Source: CAD feature listing. Evaluate the final solid. Frame: model axes, mm. Give positions to 0.01 mm unless a question says otherwise; leave off trailing zeros. Order: outer loops, then holes, each group sorted by start corner. A loop starts at its lowest first (then second) coordinate and runs counter-clockwise, first axis right, second up. Notation, with made-up numbers: M 60,77.25 L 103,77.25 A19 ccw 103,94.25 Z; hole C 87.25,-7 d10. An arc over 180 degrees is marked long. Answer in a Markdown table with one row per item. Add a question column.
(1) Section query C-C, the plane z = 0.8. Count the separate pieces of the cut face and the enclosed holes in it, plus the area to 3 significant figures.
(2) Section query A-A, the plane x = 0. Return loops of the section in (y, z).
(3) Pin query (flat end, axial travel): P1, Ø1.5, axis at x = 47.5, z = 1.5, coming from the -Y side; P2, Ø1.5, axis at y = 21, z = 3.5, coming from the -X side; P3, Ø1.5, axis at x = 48, z = 2, coming from the +Y side. Return the tip coordinate at first contact, or that it passes through.
(4) Section query D-D, the plane y = 31. Return loops of the section in (x, z).
(5) Section query B-B, the plane y = 10.16. Return loops of the section in (x, z).
(6) Material intervals for line 1 along Y through (x, z) = (-24, 1.7); line 2 along Y through (x, z) = (0, 1.2); line 3 along X through (y, z) = (3, 3.5), sorted ascending.
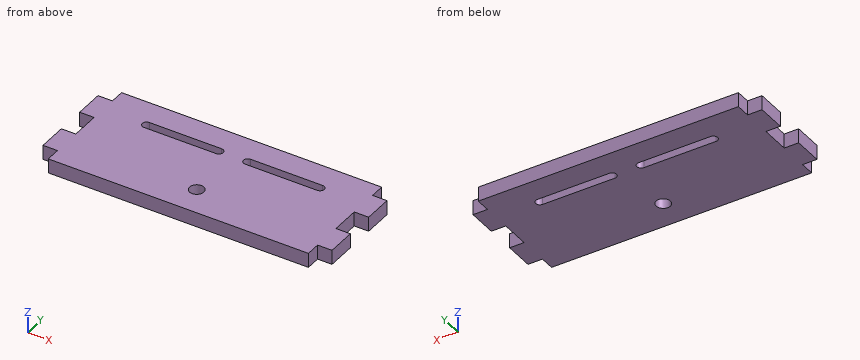
Autodesk Inventor part; units mm, degrees
ref_plane "YZ Plane" through (0, 0, 0) normal (1, 0, 0) x (0, 1, 0)
ref_plane "XZ Plane" through (0, 0, 0) normal (0, 1, 0) x (-1, 0, 0)
ref_plane "XY Plane" through (0, 0, 0) normal (0, 0, 1) x (1, 0, 0)
sketch "Sketch1" plane through (0, 0, 0) normal (0, 0, 1) x (1, 0, 0)
  line L0 (45.72, 0) -> (45.72, 40.64)
  line L1 (45.72, 40.64) -> (-45.72, 40.64)
  line L2 (-45.72, 40.64) -> (-45.72, 9.301)
  line L3 (-45.72, 5.08) -> (-50.8, 5.08)
  line L4 (-50.8, 5.08) -> (-50.8, 15.24)
  line L5 (-50.8, 15.24) -> (-45.72, 15.24)
  line L6 (-45.72, 15.24) -> (-45.72, 5.08)
  line L7 (-45.72, 25.4) -> (-50.8, 25.4)
  line L8 (-50.8, 25.4) -> (-50.8, 35.56)
  line L9 (-50.8, 35.56) -> (-45.72, 35.56)
  line L10 (-45.72, 35.56) -> (-45.72, 25.4)
  line L11 (-45.72, 45.72) -> (-50.8, 45.72)
  line L12 (-50.8, 45.72) -> (-50.8, 55.88)
  line L13 (-50.8, 55.88) -> (-45.72, 55.88)
  line L14 (-45.72, 55.88) -> (-45.72, 45.72)
  line L15 (0, 40.64) -> (0, 0) construction
  line L16 (45.72, 40.64) -> (45.72, 0)
  line L17 (45.72, 5.08) -> (50.8, 5.08)
  line L18 (50.8, 5.08) -> (50.8, 15.24)
  line L19 (50.8, 15.24) -> (45.72, 15.24)
  line L20 (45.72, 15.24) -> (45.72, 5.08)
  line L21 (45.72, 25.4) -> (50.8, 25.4)
  line L22 (50.8, 25.4) -> (50.8, 35.56)
  line L23 (50.8, 35.56) -> (45.72, 35.56)
  line L24 (45.72, 35.56) -> (45.72, 25.4)
  line L25 (45.72, 45.72) -> (50.8, 45.72)
  line L26 (50.8, 45.72) -> (50.8, 55.88)
  line L27 (50.8, 55.88) -> (45.72, 55.88)
  line L28 (45.72, 55.88) -> (45.72, 45.72)
  line L29 (-45.72, 5.08) -> (-45.72, 0)
  line L30 (-45.72, 0) -> (45.72, 0)
  line L31 (45.72, 40.64) -> (-45.72, 40.64)
  line L32 (-45.72, 40.64) -> (-45.72, 0)
  line L33 (-45.72, 0) -> (45.72, 0)
  line L34 (45.72, 0) -> (45.72, 40.64)
  dimension "d0" = 91.44
  dimension "d2" = 10.16
  dimension "d3" = 5.08
  dimension "d7" = 20.32
  dimension "d14" = 5.08
  dimension "d15" = 40.64
extrude "Extrusion2" add sketch "Sketch1" along normal blind 5.08 contours L30 L29 L6 L2 L1 L0 | L0 L19 L18 L17 | L3 L4 L5 L2 L6 | L0 L23 L22 L21 | L7 L8 L9 L2
sketch "Sketch4" plane through (0, 0, 5.08) normal (0, 0, 1) x (1, 0, 0)
  line L0 (45.72, 40.64) -> (-45.72, 40.64) construction
  line L1 (-30.48, 30.48) -> (-5.08, 30.48)
  line L2 (-30.48, 28.98) -> (-5.08, 28.98)
  line L3 (-5.08, 31.98) -> (-30.48, 31.98)
  arc A0 (-30.48, 31.98) -> (-30.48, 28.98) centre (-30.48, 30.48) ccw
  arc A1 (-5.08, 28.98) -> (-5.08, 31.98) centre (-5.08, 30.48) ccw
  line L4 (30.48, 30.48) -> (5.08, 30.48)
  line L5 (30.48, 28.98) -> (5.08, 28.98)
  line L6 (5.08, 31.98) -> (30.48, 31.98)
  arc A2 (30.48, 28.98) -> (30.48, 31.98) centre (30.48, 30.48) ccw
  arc A3 (5.08, 31.98) -> (5.08, 28.98) centre (5.08, 30.48) ccw
  line L7 (-50.8, 25.4) -> (-45.72, 25.4)
  line L8 (-45.72, 25.4) -> (-45.72, 15.24)
  line L9 (-45.72, 15.24) -> (-50.8, 15.24)
  line L10 (-50.8, 15.24) -> (-50.8, 5.08)
  line L11 (-50.8, 5.08) -> (-45.72, 5.08)
  line L12 (-45.72, 5.08) -> (-45.72, 0)
  line L13 (-45.72, 0) -> (45.72, 0)
  line L14 (45.72, 0) -> (45.72, 5.08)
  line L15 (45.72, 5.08) -> (50.8, 5.08)
  line L16 (50.8, 5.08) -> (50.8, 15.24)
  line L17 (50.8, 15.24) -> (45.72, 15.24)
  line L18 (45.72, 15.24) -> (45.72, 25.4)
  line L19 (45.72, 25.4) -> (50.8, 25.4)
  line L20 (50.8, 25.4) -> (50.8, 35.56)
  line L21 (50.8, 35.56) -> (45.72, 35.56)
  line L22 (45.72, 35.56) -> (45.72, 40.64)
  line L23 (45.72, 40.64) -> (-45.72, 40.64)
  line L24 (-45.72, 40.64) -> (-45.72, 35.56)
  line L25 (-45.72, 35.56) -> (-50.8, 35.56)
  line L26 (-50.8, 35.56) -> (-50.8, 25.4)
  line L27 (0, 40.64) -> (0, 0) construction
  circle A4 centre (0, 10.16) radius 2.5
  point P0 (-17.78, 30.48)
  point P1 (17.78, 30.48)
  point P2 (17.78, 30.48)
  dimension "d25" = 3
  dimension "d26" = 25.4
  dimension "d32" = 17.78
  dimension "d33" = 17.78
  dimension "d34" = 25.4
  dimension "d35" = 10.16
  dimension "d36" = 1.5
  dimension "d37" = 1.5
  dimension "d38" = 5
  dimension "d39" = 10.16
extrude "Extrusion5" cut sketch "Sketch4" against normal blind 25.4 contours A0 L3 A1 L2 | L5 A3 L6 A2 | A4
equation "\"d7\" = 2 * d2"
equation "\"d34\" = d26"
equation "\"d36\" = 0.5 * d25"
equation "\"d37\" = d36"
equation "\"d39\" = d35"
properties part number "EndPulleyMount" material "Wood (Birch)"
Values follow:
| question | item | result |
|---|---|---|
| 1 | separate pieces | 1 |
| 1 | enclosed holes | 3 |
| 1 | area | 3,740 mm² |
| 2 | outline | M 0,0 L 7.66,0 L 7.66,5.08 L 0,5.08 Z; M 12.66,0 L 40.64,0 L 40.64,5.08 L 12.66,5.08 Z |
| 3 | P1 | stops at y = 5.08 |
| 3 | P2 | stops at x = -45.72 |
| 3 | P3 | stops at y = 35.56 |
| 4 | outline | M -50.8,0 L -31.89,0 L -31.89,5.08 L -50.8,5.08 Z; M -3.67,0 L 3.67,0 L 3.67,5.08 L -3.67,5.08 Z; M 31.89,0 L 50.8,0 L 50.8,5.08 L 31.89,5.08 Z |
| 5 | outline | M -50.8,0 L -2.5,0 L -2.5,5.08 L -50.8,5.08 Z; M 2.5,0 L 50.8,0 L 50.8,5.08 L 2.5,5.08 Z |
| 6 | line 1 | y = 0 to 28.98, 31.98 to 40.64 |
| 6 | line 2 | y = 0 to 7.66, 12.66 to 40.64 |
| 6 | line 3 | x = -45.72 to 45.72 |
